Read the model definition and answer for the solid it produces. Units are mm, in the model's axes. Round coordinates to 2 decimals unless told otherwise and drop trailing zeros. Order: outer loops, then holes, each group sorted by start corner. A loop starts at its lowest first (then second) coordinate and runs counter-clockwise, first axis right, second up. Notation, with made-up numbers: (-24, 42) - (-16, 42) arc R9 cw to (-16, 50) - close; hole circle Ø7 at (-16, -31.75). An arc over 180 degrees is marked (long way). Answer as a JSON object with one key per item and string values. Group by question number.
Q1. Given pin 1 Ø23 at (x, y) = (56.5, 19.5) entering from +Z, flat-ended and moving along its own axis, determine where the tip first touches the part or whether it passes through.
Q2. A cutting plane is placed at C-C on y = 14. Determine the outline of the cut face in (x, z).
Q3. A cutting plane is placed at A-A on x = 134.5. Determine the outline of the cut face in (y, z).
Q4. A cutting plane is placed at B-B on z = 2.7. Determine the outline of the cut face in (x, y), and give its area (3 significant figures).
Q5. A cutting plane is placed at D-D on y = 19.5. Determine the outline of the cut face in (x, z), and give its area (3 significant figures).
Q6. Consider line 1 (Y direction, x = 17.5, z = 2.65); line 2 (X direction, y = 9.5, z = 3.3); line 3 (X direction, y = 26, z = 2.35). Determine where each line is inside the solid, lowest interval first.
```python
from build123d import *

# Parameters (mm, degrees)
SKETCH_W            = 152
SKETCH_H            = 39
PAD_DEPTH           = 5
SKETCH001_R         = 14.5
POCKET_DEPTH        = 5
LINEARPATTERN_COUNT = 4
LINEARPATTERN_PITCH = 39


with BuildPart() as part:
    # Sketch → Pad (new body)
    with BuildSketch(Plane.XY):
        with Locations((76, 19.5)):
            Rectangle(SKETCH_W, SKETCH_H)
    extrude(amount=PAD_DEPTH)

    # Sketch001 → Pocket (cut)
    with BuildSketch(Plane.XY.offset(5)):
        with Locations((17.5, 19.5)):
            Circle(SKETCH001_R)
    pocket = extrude(amount=-POCKET_DEPTH, mode=Mode.SUBTRACT)

    # LinearPattern: Pocket ×4
    with Locations(*[(i * LINEARPATTERN_PITCH, 0, 0) for i in range(1, LINEARPATTERN_COUNT)]):
        add(pocket, mode=Mode.SUBTRACT)


solid = part.part
```
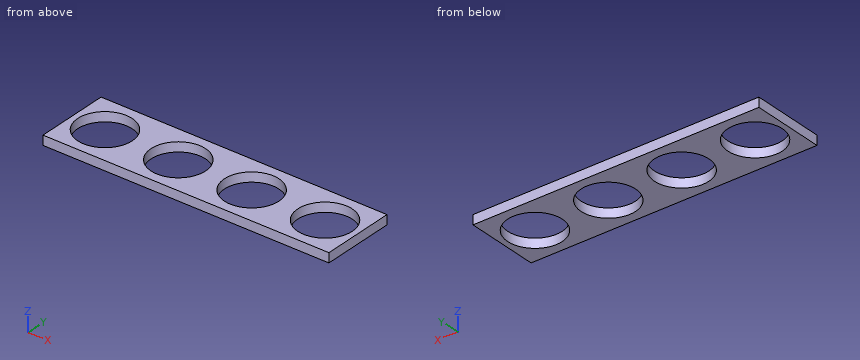
Result set:
{
 "1": {"pin 1": "passes through"},
 "2": {"outline": "(0, 0) - (4.08, 0) - (4.08, 5) - (0, 5) - close; (30.92, 0) - (43.08, 0) - (43.08, 5) - (30.92, 5) - close; (69.92, 0) - (82.08, 0) - (82.08, 5) - (69.92, 5) - close; (108.92, 0) - (121.08, 0) - (121.08, 5) - (108.92, 5) - close; (147.92, 0) - (152, 0) - (152, 5) - (147.92, 5) - close"},
 "3": {"outline": "(0, 0) - (5, 0) - (5, 5) - (0, 5) - close; (34, 0) - (39, 0) - (39, 5) - (34, 5) - close"},
 "4": {"outline": "(0, 0) - (152, 0) - (152, 39) - (0, 39) - close; hole circle Ø29 at (17.5, 19.5); hole circle Ø29 at (56.5, 19.5); hole circle Ø29 at (95.5, 19.5); hole circle Ø29 at (134.5, 19.5)", "area": "3,290 mm²"},
 "5": {"outline": "(0, 0) - (3, 0) - (3, 5) - (0, 5) - close; (32, 0) - (42, 0) - (42, 5) - (32, 5) - close; (71, 0) - (81, 0) - (81, 5) - (71, 5) - close; (110, 0) - (120, 0) - (120, 5) - (110, 5) - close; (149, 0) - (152, 0) - (152, 5) - (149, 5) - close", "area": "180 mm²"},
 "6": {"line 1": "y = 0 to 5, 34 to 39", "line 2": "x = 0 to 7, 28 to 46, 67 to 85, 106 to 124, 145 to 152", "line 3": "x = 0 to 4.54, 30.46 to 43.54, 69.46 to 82.54, 108.46 to 121.54, 147.46 to 152"}
}
